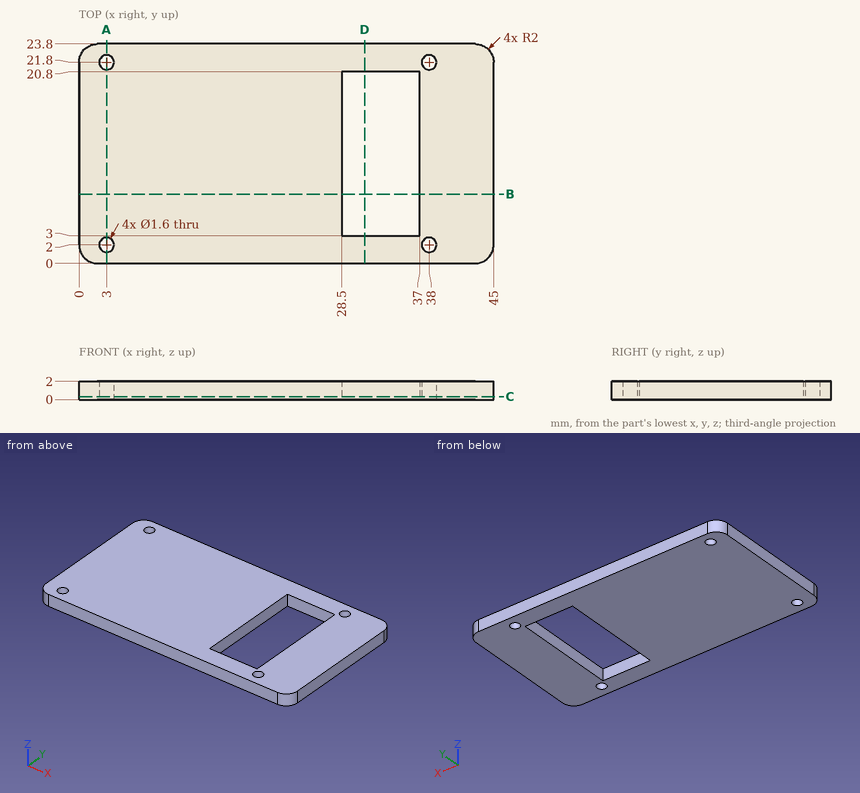
Study the drawing (mm; zero at the part's minimum x, y, z) and answer. Coordinates: 2 decimals unless noted, no trailing zeros. Write each loop counter-clockwise with the first axis right and the second up, starting at its lowest first coordinate (ties: lowest second). Pieces come first, ordered by that corner, then holes. Notation, with made-up numbers: (17, 34) - (75, 34) arc R25 ccw to (75, 59) - close; hole circle Ø3 at (26, 55). An arc over 180 degrees is marked (long way). Answer as a JSON object with one key per item and string values. Group by question number.
1. Consider L1, parallel to X at y = 7, z = 1.3; L2, parallel to Y at x = 3, z = 1; L3, parallel to Y at x = 36.5, z = 0.15. Determine where each line is inside the solid, lowest interval first. Write a range as [from, to].
2. A cutting plane is placed at D-D (x = 31). Determine the outline of the cut face in (y, z).
3. A cutting plane is placed at A-A (x = 3). Determine the outline of the cut face in (y, z), plus the area to 3 significant figures.
4. A cutting plane is placed at B-B (y = 7.5). Determine the outline of the cut face in (x, z), plus the area to 3 significant figures.
5. A cutting plane is placed at C-C (z = 0.35). Determine the outline of the cut face in (x, y), plus the area to 3 significant figures.
6. This flat-tipped pin is pushed along its axis until it touches: P1, Ø1.4, axis at x = 38, y = 21.8, coming from the -Z side. Where does it stop, or does it pass through?
Worked out:
{
 "1": {"L1": "x = [0, 28.5], [37, 45]", "L2": "y = [0, 1.2], [2.8, 21], [22.6, 23.8]", "L3": "y = [0, 3], [20.8, 23.8]"},
 "2": {"outline": "(0, 0) - (3, 0) - (3, 2) - (0, 2) - close; (20.8, 0) - (23.8, 0) - (23.8, 2) - (20.8, 2) - close"},
 "3": {"outline": "(0, 0) - (1.2, 0) - (1.2, 2) - (0, 2) - close; (2.8, 0) - (21, 0) - (21, 2) - (2.8, 2) - close; (22.6, 0) - (23.8, 0) - (23.8, 2) - (22.6, 2) - close", "area": "41.2 mm²"},
 "4": {"outline": "(0, 0) - (28.5, 0) - (28.5, 2) - (0, 2) - close; (37, 0) - (45, 0) - (45, 2) - (37, 2) - close", "area": "73.0 mm²"},
 "5": {"outline": "(0, 2) arc R2 ccw to (2, 0) - (43, 0) arc R2 ccw to (45, 2) - (45, 21.8) arc R2 ccw to (43, 23.8) - (2, 23.8) arc R2 ccw to (0, 21.8) - close; hole circle Ø1.6 at (3, 2); hole circle Ø1.6 at (3, 21.8); hole (28.5, 3) - (37, 3) - (37, 20.8) - (28.5, 20.8) - close; hole circle Ø1.6 at (38, 2); hole circle Ø1.6 at (38, 21.8)", "area": "908 mm²"},
 "6": {"P1": "passes through"}
}
